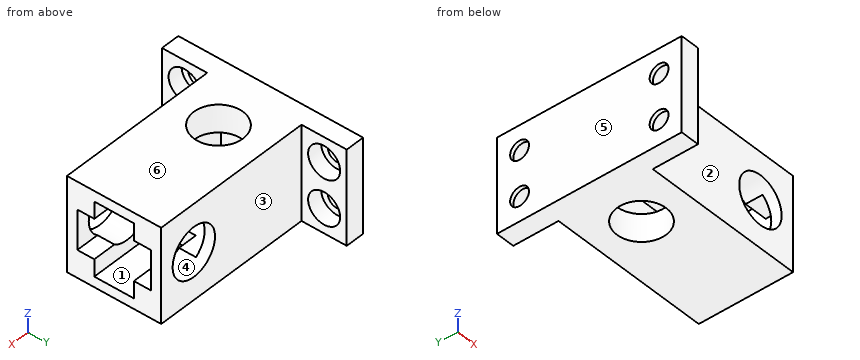
from build123d import *

# Parameters (mm, degrees)
F0_W            = 48
F0_H            = 25
F1_DEPTH        = 12.5
F2_W            = 19.5
F2_H            = 10.5
F3_DEPTH        = 44
F4_R            = 6.5
F5_DEPTH        = 25.001
F6_W            = 10.5
F6_H            = 19.5
F7_DEPTH        = 19
F8_R            = 6.5
F9_DEPTH        = 25.001
F10_W           = 12
F10_H           = 25
F11_DEPTH       = 5
F13_D           = 5
F13_CBORE_D     = 8.5
F13_CBORE_DEPTH = 4


with BuildPart() as f1:
    # F0 (on Top) → F1 (new body, symmetric)
    with BuildSketch(Plane.XY):
        with Locations((8, 0)):
            Rectangle(F0_W, F0_H)
    extrude(amount=F1_DEPTH, both=True)

    # F2 (on face) → F3 (cut)
    with BuildSketch(Plane.YZ.offset(32)):
        Rectangle(F2_W, F2_H)
    extrude(amount=-F3_DEPTH, mode=Mode.SUBTRACT)

    # F4 (on face) → F5 (cut, through all)
    with BuildSketch(Plane(origin=(0, 0, -12.5), x_dir=(1, 0, 0), z_dir=(0, 0, -1))):
        Circle(F4_R)
    extrude(amount=-F5_DEPTH, mode=Mode.SUBTRACT)

    # F6 (on face) → F7 (cut)
    with BuildSketch(Plane.YZ.offset(32)):
        Rectangle(F6_W, F6_H)
    extrude(amount=-F7_DEPTH, mode=Mode.SUBTRACT)

    # F8 (on face) → F9 (cut, through all)
    with BuildSketch(Plane.XZ.offset(12.5)):
        with Locations((22, 0)):
            Circle(F8_R)
    extrude(amount=-F9_DEPTH, mode=Mode.SUBTRACT)

    # F10 (on face) → F11 (join)
    with BuildSketch(Plane(origin=(-16, 0, 0), x_dir=(0, -1, 0), z_dir=(-1, 0, 0))):
        with Locations((-18.5, 0)):
            Rectangle(F10_W, F10_H)
        with Locations((18.5, 0)):
            Rectangle(F10_W, F10_H)
    extrude(amount=-F11_DEPTH)

    # F13 (through all)
    with Locations(Plane.YZ.offset(-11)):
        with Locations((-18.5, 6), (-18.5, -6), (18.5, 6), (18.5, -6)):
            CounterBoreHole(F13_D / 2, F13_CBORE_D / 2, F13_CBORE_DEPTH)


solid = f1.part
Build history of the part. All positions in model axes, mm. Face numbers are marked on the shaded views. A direction names the side the tool comes from. Round coordinates to 2 decimals unless told otherwise and drop trailing zeros. Order: outer loops, then holes, each group sorted by start corner. A loop starts at its lowest first (then second) coordinate and runs counter-clockwise, first axis right, second up. Notation, with made-up numbers: M -6,47 L 8,47 A12 cw 8,65 Z; hole C 86.5,5 d1. An arc over 180 degrees is marked long. Use CSV: the item, a comma, the result in double quotes. Start each with the question number.
(1) Tool access for the marked faces 1, 2 and 3: list every direction of +Z, -Z, +X, -X, +Y, -Y with a clear straight run to the whole face (end or side of a thin tool).
(2) Cut at C-C on z = 0. List the corners of the cut face in (x, y), then the cut area to 4 significant figures.
(3) Cut at A-A on y = -18.5. List the corners of the cut face in (x, z), then the cut area to 3 significant figures.
(4) Drill centre lines: probe 1 along Z at (x, y) = (-15.8, -18.5); probe 2 along Z at (x, y) = (-6, -4); probe 3 along Y at (x, z) = (-0.5, 0.25). Where is each one in solid material? Low to high.
(5) Cut at D-D on x = 8.5. List the corners of the cut face in (y, z), then the cut area to 3 significant figures.
(6) Cut at B-B on x = 22. List the corners of the cut face in (y, z).
(7) Flat gauge pins, fed straight in: P1, Ø2.5, axis at y = 16.5, z = 5, coming from the +X side; P2, Ø10, axis at x = -0.5, z = -0.5, coming from the -Y side; P3, Ø11.5, axis at y = 0.5, z = -0.5, coming from the +X side; P4, Ø10, axis at x = 26, y = -19, coming from the -Z side. Where does each tip first touch, or does it go through?
(8) Mould opens along X. For the marked faces 4, 5 and 6 say: +X half, -X half, draft (parallel to the pull), parting line (faces both ways), or undercut.
Findings:
1,face 1,"+X"
1,face 2,"+Z, -Z, +X, -Y"
1,face 3,"+Z, -Z, +X, +Y"
2,outline,"M -16,-24.5 L -11,-24.5 L -11,-12.5 L 15.5,-12.5 L 15.5,-9.75 L -12,-9.75 L -12,9.75 L 15.5,9.75 L 15.5,12.5 L -11,12.5 L -11,24.5 L -16,24.5 Z; M 28.5,-12.5 L 32,-12.5 L 32,-9.75 L 28.5,-9.75 Z; M 28.5,9.75 L 32,9.75 L 32,12.5 L 28.5,12.5 Z"
2,area,"390.5 mm^2"
3,outline,"M -16,-12.5 L -11,-12.5 L -11,-10.25 L -15,-10.25 L -15,-8.5 L -16,-8.5 Z; M -16,-3.5 L -15,-3.5 L -15,-1.75 L -11,-1.75 L -11,1.75 L -15,1.75 L -15,3.5 L -16,3.5 Z; M -16,8.5 L -15,8.5 L -15,10.25 L -11,10.25 L -11,12.5 L -16,12.5 Z"
3,area,"47.0 mm^2"
4,probe 1,"z = -12.5 to -8.5, -3.5 to 3.5, 8.5 to 12.5"
4,probe 2,"z = -12.5 to -5.25, 5.25 to 12.5"
4,probe 3,"y = -12.5 to -9.75, 9.75 to 12.5"
5,outline,"M -12.5,-12.5 L 12.5,-12.5 L 12.5,12.5 L -12.5,12.5 Z; hole M -9.75,-5.25 L 9.75,-5.25 L 9.75,5.25 L -9.75,5.25 Z"
5,area,"420 mm^2"
6,outline,"M -12.5,-12.5 L 12.5,-12.5 L 12.5,-6.5 L 5.25,-6.5 L 5.25,-9.75 L -5.25,-9.75 L -5.25,-6.5 L -12.5,-6.5 Z; M -12.5,6.5 L -5.25,6.5 L -5.25,9.75 L 5.25,9.75 L 5.25,6.5 L 12.5,6.5 L 12.5,12.5 L -12.5,12.5 Z"
7,P1,"stops at x = -15"
7,P2,"stops at y = -12.5"
7,P3,"stops at x = 13"
7,P4,"passes through"
8,face 4,"undercut"
8,face 5,"-X half"
8,face 6,"draft"
